```python
from build123d import *

# Parameters (mm, degrees)
SKETCH_1_R      = 6
SKETCH_1_R_2    = 4
EXTRUDE_1_DEPTH = 2
CHAMFER_1_SIZE  = 0.2


with BuildPart() as part:
    # 草图1 → 拉伸1 (new body)
    with BuildSketch(Plane.XY):
        Circle(SKETCH_1_R)
        Circle(SKETCH_1_R_2, mode=Mode.SUBTRACT)
    extrude(amount=EXTRUDE_1_DEPTH)

    # 倒角1
    chamfer_1_edges = [part.edges().sort_by_distance(p)[0] for p in [
        (-6, 0, 0),
        (-6, 0, 2),
        (-4, 0, 0),
        (-4, 0, 2),
    ]]
    chamfer(chamfer_1_edges, length=CHAMFER_1_SIZE)


solid = part.part
```
Can you work these out from the model? Positions are in its coordinate system, mm. Give positions to 0.01 mm unless a question says otherwise; leave off trailing zeros. Loops run counter-clockwise (first coordinate to the right, second up) from the corner with the lowest first, then second, coordinate; pieces in that order, holes last. Notation, with made-up numbers: M 1.25,40 L 57.25,40 A7 cw 57.25,44 Z; hole C 16,69.25 d11. An arc over 180 degrees is marked long. Use CSV: the item, a comma, the result in double quotes. Start each with the question number.
1. Imagine slicing it at C-C, the plane z = 1.5. Write out the boundary of the cut face in (x, y), plus the area to 3 significant figures.
2. For P1, Ø1, axis at x = 2, z = 0, coming from the -Y side, with a flat end and sliding along its axis, tell me the tip position at first contact or that it passes through.
3. If I drill on L1, parallel to Y at x = 0, z = 0.9; L2, parallel to Y at x = -2, z = 1.3; L3, parallel to X at y = 2.25, z = 0.9, over which ranges is the centre line in solid material (lowest first)?
4. Imagine slicing it at A-A, the plane x = 0. Write out the boundary of the cut face in (y, z).
5. If we mould it in two halves opening along Y, with no side actions, what happens to faces 1 (the face through (4, 2, 0)), 2 (the face through (-6, 0, 1)), 3 (the face through (-0.867, -3.905, 0.989))? For each: released by +Y, released by -Y, zero draft, split by the parting line, or undercut.
Response values:
1,outline,"C 0,0 d12; hole C 0,0 d8"
1,area,"62.8 mm^2"
2,P1,"y = -5.8"
3,L1,"-6 to -4, 4 to 6"
3,L2,"-5.66 to -3.46, 3.46 to 5.66"
3,L3,"-5.56 to -3.31, 3.31 to 5.56"
4,outline,"M -6,0.2 L -5.8,0 L -4.2,0 L -4,0.2 L -4,1.8 L -4.2,2 L -5.8,2 L -6,1.8 Z; M 4,0.2 L 4.2,0 L 5.8,0 L 6,0.2 L 6,1.8 L 5.8,2 L 4.2,2 L 4,1.8 Z"
5,face 1,"zero draft"
5,face 2,"split by the parting line"
5,face 3,"undercut"
